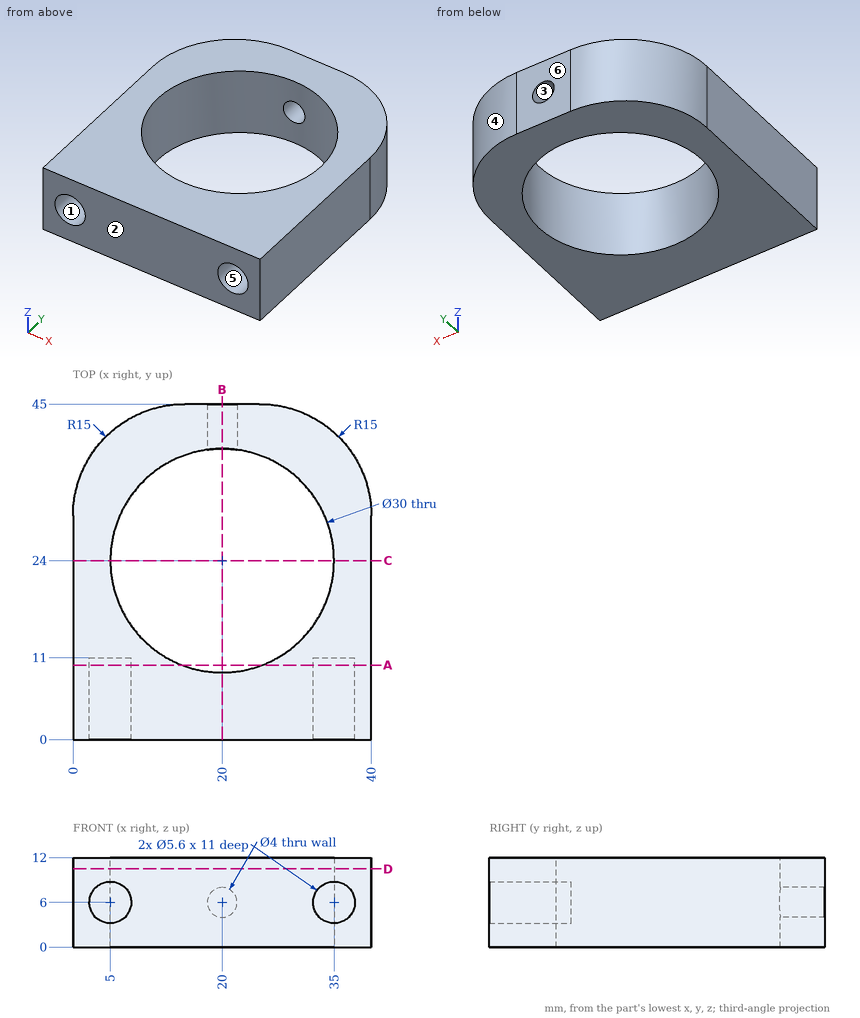
Part print with two shaded views. Sizes in mm from the minimum x, y, z corner. A direction names the side the tool comes from. Round coordinates to 2 decimals unless told otherwise and drop trailing zeros. Write each loop counter-clockwise with the first axis right and the second up, starting at its lowest first coordinate (ties: lowest second). Pieces come first, ordered by that corner, then holes. Notation, with made-up numbers: (-14, -2.75) - (28, -2.75) arc R15 ccw to (28, 3.25) - close; hole circle Ø5 at (34.25, -34). An arc over 180 degrees is marked (long way). Use CSV: the item, a comma, the result in double quotes.
Item 1: Wall check: L1, parallel to X at y = 2.75, z = 6; L2, parallel to X at y = 7, z = 5.25; L3, parallel to Z at x = 35, y = 5. Give the ranges that are in metal, low to high.
Results list:
L1,"x = 0 to 2.2, 7.8 to 32.2, 37.8 to 40"
L2,"x = 0 to 2.3, 7.7 to 32.3, 37.7 to 40"
L3,"z = 0 to 3.2, 8.8 to 12"
Item 2: Flat gauge pins, fed straight in: P1, Ø1.7, axis at x = 35, z = 7, coming from the -Y side; P2, Ø5, axis at x = 31.5, z = 6, coming from the +Y side; P3, Ø1, axis at x = 27, z = 6, coming from the +Y side. Where does each tip first touch, or does it go through?
Results list:
P1,"stops at y = 11"
P2,"stops at y = 44.46"
P3,"stops at y = 44.92"
Item 3: Pull direction X, two halves, no side cores. Call the marked faces 4, 5 and 6: pulls with the +X half, pulls with the -X half, needs draft (parallel to the pull), parting line crosses it, or undercut.
Results list:
face 4,"pulls with the +X half"
face 5,"undercut"
face 6,"needs draft"
Item 4: Slice it at D-D, the plane z = 10.5. Write the cut outline in (x, y), then the cut area to 3 significant figures.
Results list:
outline,"(0, 0) - (40, 0) - (40, 30) arc R15 ccw to (25, 45) - (15, 45) arc R15 ccw to (0, 30) - close; hole circle Ø30 at (20, 24)"
area,"997 mm²"
Item 5: Tool access for the marked faces 1, 2 and 3: list every direction of +Z, -Z, +X, -X, +Y, -Y with a clear straight run to the whole face (end or side of a thin tool).
Results list:
face 1,"-Y"
face 2,"+Z, -Z, +X, -X, -Y"
face 3,"+Y"
Item 6: Slice it at C-C, the plane y = 24. Write the cut outline in (x, z), then the cut area to 3 significant figures.
Results list:
outline,"(0, 0) - (5, 0) - (5, 12) - (0, 12) - close; (35, 0) - (40, 0) - (40, 12) - (35, 12) - close"
area,"120 mm²"
Item 7: Slice it at B-B, the plane x = 20. Write the cut outline in (y, z), then the cut area to 3 significant figures.
Results list:
outline,"(0, 0) - (9, 0) - (9, 12) - (0, 12) - close; (39, 0) - (45, 0) - (45, 4) - (39, 4) - close; (39, 8) - (45, 8) - (45, 12) - (39, 12) - close"
area,"156 mm²"
Item 8: Slice it at A-A, the plane y = 10. Write the cut outline in (x, z).
Results list:
outline,"(0, 0) - (14.61, 0) - (14.61, 12) - (0, 12) - close; (25.39, 0) - (40, 0) - (40, 12) - (25.39, 12) - close; hole circle Ø5.6 at (5, 6); hole circle Ø5.6 at (35, 6)"
